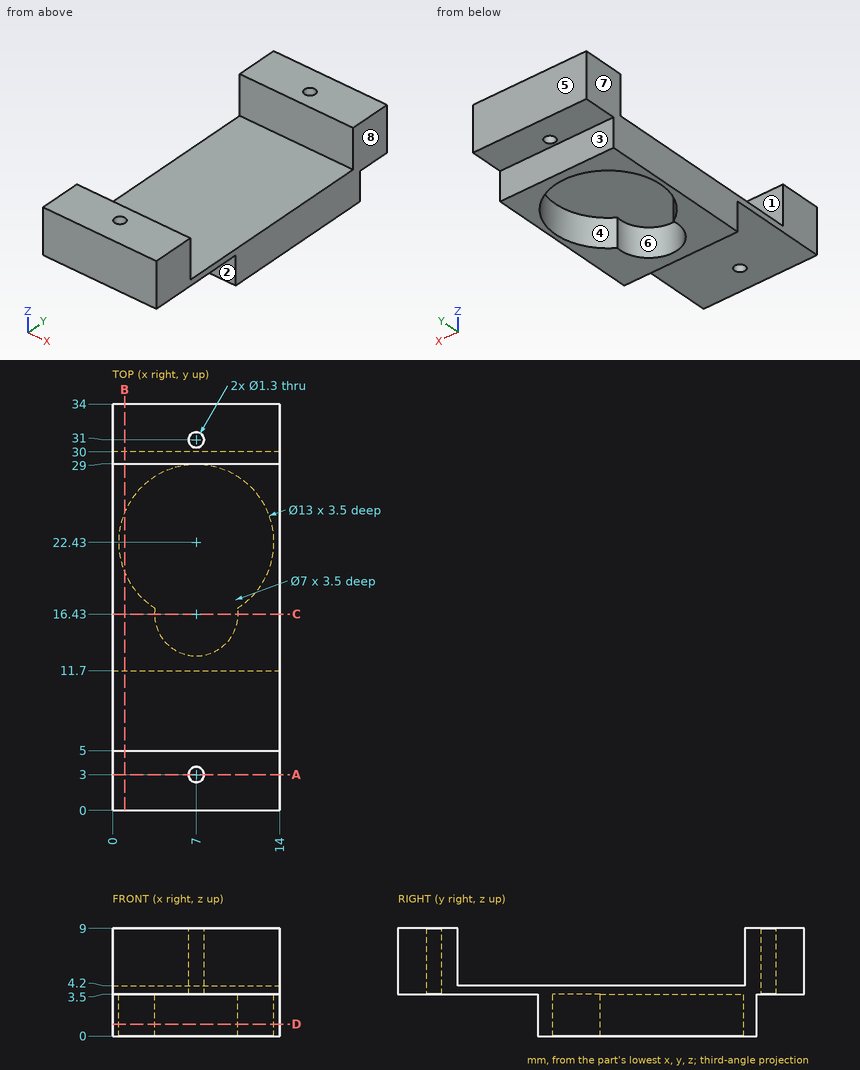
The drawing under review shows one solid part. Ordinate dimensions are in mm from its lowest x, y, z. A direction names the side the tool comes from. Coordinates: 2 decimals unless noted, no trailing zeros. Write each loop counter-clockwise with the first axis right and the second up, starting at its lowest first coordinate (ties: lowest second). Pieces come first, ordered by that corner, then holes. Notation, with made-up numbers: (-32.5, -25) - (11.5, -25) arc R35 ccw to (11.5, 9) - close; hole circle Ø6 at (-18, -15.5). An arc over 180 degrees is marked (long way). Answer in a Markdown table with one row per item. Add a question column.
Q1. We need section A-A, the plane y = 3. State the section outline as (x, z) points.
Q2. For P1, Ø4.5, axis at x = 3.5, y = 32.5, coming from the -Z side; P2, Ø5.5, axis at x = 7, y = 16.43, coming from the +Z side; P3, Ø1.1, axis at x = 8, z = 2, coming from the +Y side, all flat-tipped, find the tip position at first contact; note any pin that passes through.
Q3. Draft analysis for pull direction X (two halves, no side actions). For the marked faces 5, 6, 7 and 8, state which applies: +X half, -X half, draft (parallel to the pull), parting line (faces both ways), or undercut.
Q4. Tool access review of the marked faces 1, 2, 3 and 4: name each direction out of +Z, -Z, +X, -X, +Y, -Y from which nothing blocks a thin tool from reaching the whole face with its end or side.
Q5. For probe 1 along X at (y, z) = (16.43, 1.8); probe 2 along X at (y, z) = (3, 5.5); probe 3 along Y at (x, z) = (7, 1.75), list the stretches that pass through material, from the lowest coordinate up.
Q6. We need section C-C, the plane y = 16.43. State the section outline as (x, z) points.
Q7. We need section B-B, the plane x = 1. State the section outline as (y, z) points.
Q8. We need section D-D, the plane z = 1. State the section outline as (x, y) points.
Answer list:
| question | item | result |
|---|---|---|
| 1 | outline | (0, 3.5) - (6.35, 3.5) - (6.35, 9) - (0, 9) - close; (7.65, 3.5) - (14, 3.5) - (14, 9) - (7.65, 9) - close |
| 2 | P1 | stops at z = 3.5 |
| 2 | P2 | stops at z = 4.2 |
| 2 | P3 | stops at y = 30 |
| 3 | face 5 | draft |
| 3 | face 6 | undercut |
| 3 | face 7 | -X half |
| 3 | face 8 | +X half |
| 4 | face 1 | +Z, +X, -X |
| 4 | face 2 | -Z, +X, -X, -Y |
| 4 | face 3 | -Z, +X, -X, +Y |
| 4 | face 4 | -Z |
| 5 | probe 1 | x = 0 to 3.5, 10.5 to 14 |
| 5 | probe 2 | x = 0 to 6.35, 7.65 to 14 |
| 5 | probe 3 | y = 11.7 to 12.93, 28.93 to 30 |
| 6 | outline | (0, 0) - (3.5, 0) - (3.5, 3.5) - (10.5, 3.5) - (10.5, 0) - (14, 0) - (14, 4.2) - (0, 4.2) - close |
| 7 | outline | (0, 3.5) - (11.7, 3.5) - (11.7, 0) - (19.93, 0) - (19.93, 3.5) - (24.93, 3.5) - (24.93, 0) - (30, 0) - (30, 3.5) - (34, 3.5) - (34, 9) - (29, 9) - (29, 4.2) - (5, 4.2) - (5, 9) - (0, 9) - close |
| 8 | outline | (0, 11.7) - (14, 11.7) - (14, 30) - (0, 30) - close; hole (3.54, 16.93) arc R3.5 ccw (long way) to (10.46, 16.93) arc R6.5 ccw (long way) to start |
